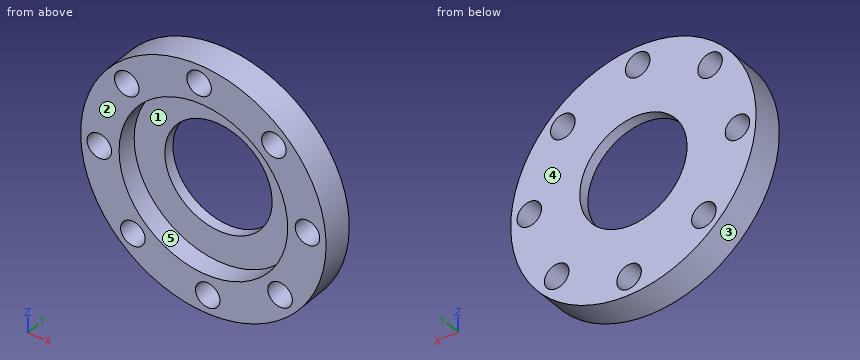
from build123d import *

# Parameters (mm, degrees)
SKETCH1_R           = 40
BOSS_EXTRUDE1_DEPTH = 10
SKETCH3_R           = 27.5
CUT_EXTRUDE2_DEPTH  = 6.5
SKETCH4_R           = 17.5
CUT_EXTRUDE3_DEPTH  = 58.445626465
SKETCH5_R           = 4
CUT_EXTRUDE4_DEPTH  = 58.445626465


with BuildPart() as part:
    # Sketch1 → Boss-Extrude1 (new body)
    with BuildSketch(Plane(origin=(0, 0, 0), x_dir=(1, 0, 0), z_dir=(0, 1, 0))):
        with Locations(Location((0, 0, 0), (0, 0, 270))):
            Circle(SKETCH1_R)
    extrude(amount=BOSS_EXTRUDE1_DEPTH)

    # Sketch3 → Cut-Extrude2 (cut)
    with BuildSketch(Plane.XZ):
        with Locations(Location((0, 0, 0), (0, 0, 270))):
            Circle(SKETCH3_R)
    extrude(amount=-CUT_EXTRUDE2_DEPTH, mode=Mode.SUBTRACT)

    # Sketch4 → Cut-Extrude3 (cut, through all)
    with BuildSketch(Plane(origin=(0, 10, 0), x_dir=(1, 0, 0), z_dir=(0, 1, 0))):
        with Locations(Location((0, 0, 0), (0, 0, 270))):
            Circle(SKETCH4_R)
    extrude(amount=-CUT_EXTRUDE3_DEPTH, mode=Mode.SUBTRACT)

    # Sketch5 → Cut-Extrude4 (cut, through all)
    with BuildSketch(Plane.XZ):
        with Locations(Location((-25, 23, 0), (0, 0, 270))):
            Circle(SKETCH5_R)
        with Locations(Location((-1.414213562, 33.941125497, 0), (0, 0, 270))):
            Circle(SKETCH5_R)
        with Locations(Location((23, 25, 0), (0, 0, 270))):
            Circle(SKETCH5_R)
        with Locations(Location((33.941125497, 1.414213562, 0), (0, 0, 270))):
            Circle(SKETCH5_R)
        with Locations(Location((25, -23, 0), (0, 0, 270))):
            Circle(SKETCH5_R)
        with Locations(Location((1.414213562, -33.941125497, 0), (0, 0, 270))):
            Circle(SKETCH5_R)
        with Locations(Location((-23, -25, 0), (0, 0, 270))):
            Circle(SKETCH5_R)
        with Locations(Location((-33.941125497, -1.414213562, 0), (0, 0, 270))):
            Circle(SKETCH5_R)
    extrude(amount=-CUT_EXTRUDE4_DEPTH, mode=Mode.SUBTRACT)


solid = part.part
CAD build for the part. Positions are in the model's coordinates, mm. Face numbers are marked on the shaded views. A direction names the side the tool comes from. Round coordinates to 2 decimals unless told otherwise and drop trailing zeros. Write each loop counter-clockwise with the first axis right and the second up, starting at its lowest first coordinate (ties: lowest second). Pieces come first, ordered by that corner, then holes. Notation, with made-up numbers: (57, -26.75) -> (67, -26.75) arc R33 ccw to (67, 6.25) -> close; hole circle Ø7 at (21.25, 82). An arc over 180 degrees is marked (long way). Answer as a JSON object with one key per item and string values.
(1) Two-plate mould, pull along X, no slides. Class the marked faces 3, 4 and 5: +X half, -X half, draft (parallel to the pull), parting line (faces both ways), or undercut.
Reported:
{"face 3": "parting line", "face 4": "draft", "face 5": "undercut"}
(2) Probe probe 1 along Z at (x, y) = (-22, 2.25); probe 2 along Z at (x, y) = (-20.5, 5.25); probe 3 along X at (y, z) = (8, 23). List the from-to ranges inside material, lowest first. Write a range as [from, to].
Reported:
{"probe 1": "z = [-33.41, -28.87], [-21.13, -16.5], [16.5, 20.35], [25.65, 33.41]", "probe 2": "z = [-34.35, -28.12], [-21.88, -18.33], [18.33, 34.35]", "probe 3": "x = [-32.73, -29], [-21, 19.54], [26.46, 32.73]"}
(3) Which spindle directions (+Z, -Z, +X, -X, +Y, -Y) get a long thin tool onto all of the face, cutting with end or side? Do the marked faces 1 and 2. Say none if no direction does.
Reported:
{"face 1": "-Y", "face 2": "+Z, -Z, +X, -X, -Y"}
(4) Band-saw the part on A-A, the plane x = 23. List the corners of the cut face in (y, z), then the cut area to 3 significant figures.
Reported:
{"outline": "(0, -32.73) -> (10, -32.73) -> (10, -26.46) -> (0, -26.46) -> close; (0, -19.54) -> (10, -19.54) -> (10, 21) -> (0, 21) -> (0, 15.07) -> (6.5, 15.07) -> (6.5, -15.07) -> (0, -15.07) -> close; (0, 29) -> (10, 29) -> (10, 32.73) -> (0, 32.73) -> close", "area": "309 mm^2"}
(5) Band-saw the part on D-D, the plane z = 25. List the corners of the cut face in (x, y).
Reported:
{"outline": "(-31.22, 0) -> (-28.46, 0) -> (-28.46, 10) -> (-31.22, 10) -> close; (-21.54, 0) -> (-11.46, 0) -> (-11.46, 6.5) -> (11.46, 6.5) -> (11.46, 0) -> (19, 0) -> (19, 10) -> (-21.54, 10) -> close; (27, 0) -> (31.22, 0) -> (31.22, 10) -> (27, 10) -> close"}
(6) Band-saw the part on C-C, the plane x = 0. List the corners of the cut face in (y, z), then the cut area to 3 significant figures.
Reported:
{"outline": "(0, -40) -> (10, -40) -> (10, -37.68) -> (0, -37.68) -> close; (0, -30.2) -> (10, -30.2) -> (10, -17.5) -> (6.5, -17.5) -> (6.5, -27.5) -> (0, -27.5) -> close; (0, 27.5) -> (6.5, 27.5) -> (6.5, 17.5) -> (10, 17.5) -> (10, 30.2) -> (0, 30.2) -> close; (0, 37.68) -> (10, 37.68) -> (10, 40) -> (0, 40) -> close", "area": "170 mm^2"}
(7) Pin check, flat tips, straight feed: P1, Ø13, axis at x = -23, z = -25, coming from the -Y side; P2, Ø4, axis at y = 3.5, z = -28.5, coming from the -X side; P3, Ø1.5, axis at x = 11, y = 6.5, coming from the +Z side; P4, Ø5, axis at x = 15, y = 7.5, coming from the -Z side. Stop position of each tip, or through.
Reported:
{"P1": "stops at y = 0", "P2": "stops at x = -29.96", "P3": "stops at z = 38.66", "P4": "stops at z = -38"}
(8) Band-saw the part on B-B, the plane z = 11. List the corners of the cut face in (x, y), then the cut area to 3 significant figures.
Reported:
{"outline": "(-38.46, 0) -> (-25.2, 0) -> (-25.2, 6.5) -> (-13.61, 6.5) -> (-13.61, 10) -> (-38.46, 10) -> close; (13.61, 6.5) -> (25.2, 6.5) -> (25.2, 0) -> (38.46, 0) -> (38.46, 10) -> (13.61, 10) -> close", "area": "346 mm^2"}
